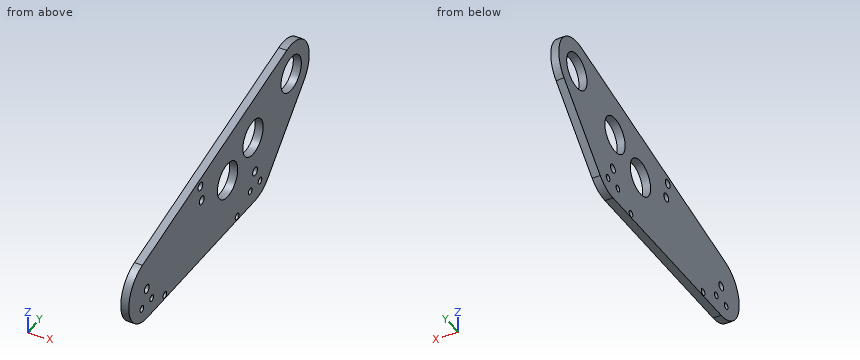
from build123d import *

# Parameters (mm, degrees)
BOSS_EXTRUDE1_DEPTH     = 6.35
F_1_1_DIAMETER_HOLE1_D  = 28.575
F_1_4_CLEARANCE_HOLE1_D = 6.7564
F_1_4_20_TAPPED_HOLE1_D = 5.1054
F_1_4_CLEARANCE_HOLE2_D = 6.7564
F_10_CLEARANCE_HOLE1_D  = 5.1054


with BuildPart() as part:
    # Sketch2 → Boss-Extrude1 (new body)
    with BuildSketch(Plane(origin=(0, 0, 0), x_dir=(0, 0, -1), z_dir=(1, 0, 0))):
        with BuildLine():
            Line((68.760512242, -32.839487758), (17.960512242, 17.960512242))
            ThreePointArc((17.960512242, 17.960512242), (-12.514549901, 22.103077632), (-24.641619504, -6.160404876))
            Line((-24.641619504, -6.160404876), (26.158380496, -209.360404876))
            ThreePointArc((26.158380496, -209.360404876), (53.903454898, -228.40969194), (76.2, -203.2))
            Line((76.2, -203.2), (76.2, -50.8))
            ThreePointArc((76.2, -50.8), (74.266540126, -41.079840818), (68.760512242, -32.839487758))
        make_face()
    extrude(amount=BOSS_EXTRUDE1_DEPTH)

    # 1 (1) Diameter Hole1 (through all)
    with Locations(Plane(origin=(6.35, 0, 0), x_dir=(0, 0, -1), z_dir=(1, 0, 0))):
        with Locations((0, 0), (19.546451191, -53.703433278), (32.577418652, -89.50572213)):
            Hole(F_1_1_DIAMETER_HOLE1_D / 2)

    # 1/4 Clearance Hole1 (through all)
    with Locations(Plane(origin=(6.35, 0, 0), x_dir=(0, 0, -1), z_dir=(1, 0, 0))):
        with Locations((50.8, -50.8), (50.8, -203.2), (12.320809752, -127.828401175)):
            Hole(F_1_4_CLEARANCE_HOLE1_D / 2)

    # 1/4-20 Tapped Hole1 (through all)
    with Locations(Plane.ZY):
        with Locations((-63.5, -57.7088), (-63.5, -43.8912), (-63.5, -210.1088), (-63.5, -196.2912)):
            Hole(F_1_4_20_TAPPED_HOLE1_D / 2)

    # 1/4 Clearance Hole2 (through all)
    with Locations(Plane.ZY):
        with Locations((-25.535413776, -125.85644657)):
            Hole(F_1_4_CLEARANCE_HOLE2_D / 2)

    # #10 Clearance Hole1 (through all)
    with Locations(Plane.ZY):
        with Locations((-73.025, -76.2), (-73.025, -177.8)):
            Hole(F_10_CLEARANCE_HOLE1_D / 2)


solid = part.part
Input: part model. Units: mm. Frame: model coordinates. Give positions to 0.01 mm unless a question says otherwise; leave off trailing zeros. Order: outer loops, then holes, each group sorted by start corner. A loop starts at its lowest first (then second) coordinate and runs counter-clockwise, first axis right, second up.
Q1. Section B-B on z = 0. Output: boundary loops of the cut face in (x, y), and give its area (3 significant figures).
Checked values:
outline: (0, -104.73) - (6.35, -104.73) - (6.35, -14.29) - (0, -14.29) - close; (0, 14.29) - (6.35, 14.29) - (6.35, 25.4) - (0, 25.4) - close
area: 645 mm2
Q2. Section A-A on y = 0. Output: boundary loops of the cut face in (x, z).
Checked values:
outline: (0, -35.92) - (6.35, -35.92) - (6.35, -14.29) - (0, -14.29) - close; (0, 14.29) - (6.35, 14.29) - (6.35, 25.4) - (0, 25.4) - close
Q3. Section D-D on x = 1. State how many separate pieces and enclosed holes the cut face has, and give its area (3 significant figures).
Checked values:
separate pieces: 1
enclosed holes: 13
area: 14,700 mm2
Q4. Section C-C on z = -50.8. Output: boundary loops of the cut face in (x, y).
Checked values:
outline: (0, -228.6) - (6.35, -228.6) - (6.35, -206.58) - (0, -206.58) - close; (0, -199.82) - (6.35, -199.82) - (6.35, -54.18) - (0, -54.18) - close; (0, -47.42) - (6.35, -47.42) - (6.35, -14.88) - (0, -14.88) - close
Q5. Ray query, probe 1 along Y at (x, z) = (4.5, -50.8); probe 2 along Y at (x, z) = (3.5, -63.5); probe 3 along Z at (x, y) = (2, -177.8). Return the intervals inside material, ascending.
Checked values:
probe 1: y = -228.6 to -206.58, -199.82 to -54.18, -47.42 to -14.88
probe 2: y = -225.2 to -212.66, -207.56 to -198.84, -193.74 to -60.26, -55.16 to -46.44, -41.34 to -27.58
probe 3: z = -76.2 to -75.58, -70.47 to -18.27
Q6. Contact query for flat-ended pins moving along their axis: pin 1 Ø2 at (x, z) = (3.5, -36.5) entering from +Y; pin 2 Ø6 at (y, z) = (-210.11, -63.5) entering from -X; pin 3 Ø2 at (x, y) = (3, -48) entering from -Z. Output: stop coordinate, or through.
Checked values:
pin 1: stops at y = 0.42
pin 2: stops at x = 0
pin 3: stops at z = -76.14
